Geometry check sheet. Reference: the model listing, model coordinates, mm. Round coordinates to 2 decimals unless told otherwise and drop trailing zeros. Order: outer loops, then holes, each group sorted by start corner. A loop starts at its lowest first (then second) coordinate and runs counter-clockwise, first axis right, second up.
```python
from build123d import *

# Parameters (mm, degrees)
F1_DEPTH = 3.81
F2_R     = 5.9944
F3_DEPTH = 25.4
F4_R     = 25.4


with BuildPart() as f1:
    # F0 (on Front) → F1 (new body)
    with BuildSketch(Plane.XZ):
        with BuildLine():
            ThreePointArc((-77.47, 0), (-76.2, 1.27), (-74.93, 0))
            Line((-74.93, 0), (-1.27, 0))
            ThreePointArc((-1.27, 0), (0, 1.27), (1.27, 0))
            Line((1.27, 0), (12.7, 0))
            Line((12.7, 0), (12.7, 12.7))
            Line((12.7, 12.7), (-88.9, 12.7))
            Line((-88.9, 12.7), (-88.9, 0))
            Line((-88.9, 0), (-77.47, 0))
        make_face()
        with BuildLine():
            ThreePointArc((-76.2, -1.27), (-77.0980256121, -0.8980256121), (-77.47, 0))
            Line((-77.47, 0), (-88.9, 0))
            Line((-88.9, 0), (-88.9, -76.2))
            Line((-88.9, -76.2), (-76.2, -76.2))
            Line((-76.2, -76.2), (-76.2, -1.27))
        make_face()
        with BuildLine():
            Line((-1.27, 0), (-74.93, 0))
            ThreePointArc((-74.93, 0), (-75.3019743879, -0.8980256121), (-76.2, -1.27))
            Line((-76.2, -1.27), (-76.2, -76.2))
            Line((-76.2, -76.2), (-69.85, -76.2))
            Line((-69.85, -76.2), (-6.35, -76.2))
            Line((-6.35, -76.2), (-6.35, -71.12))
            ThreePointArc((-6.35, -71.12), (-7.2480256121, -68.9519743879), (-5.08, -69.85))
            Line((-5.08, -69.85), (0, -69.85))
            Line((0, -69.85), (0, -1.27))
            ThreePointArc((0, -1.27), (-0.8980256121, -0.8980256121), (-1.27, 0))
        make_face()
        with BuildLine():
            ThreePointArc((-68.58, -69.85), (-68.9519743879, -70.7480256121), (-69.85, -71.12))
            ThreePointArc((-69.85, -71.12), (-70.7480256121, -68.9519743879), (-68.58, -69.85))
        make_face(mode=Mode.SUBTRACT)
        with BuildLine():
            Line((0, -76.2), (0, -69.85))
            Line((0, -69.85), (-5.08, -69.85))
            ThreePointArc((-5.08, -69.85), (-5.4519743879, -70.7480256121), (-6.35, -71.12))
            Line((-6.35, -71.12), (-6.35, -76.2))
            Line((-6.35, -76.2), (0, -76.2))
        make_face()
        with BuildLine():
            Line((12.7, 0), (1.27, 0))
            ThreePointArc((1.27, 0), (0.8980256121, -0.8980256121), (0, -1.27))
            Line((0, -1.27), (0, -69.85))
            Line((0, -69.85), (0, -76.2))
            Line((0, -76.2), (12.7, -76.2))
            Line((12.7, -76.2), (12.7, 0))
        make_face()
    extrude(amount=F1_DEPTH)

    # F2 (on face) → F3 (cut)
    with BuildSketch(Plane.XZ.offset(3.81)):
        with Locations((-70.104, -31.75)):
            Circle(F2_R)
        with BuildLine():
            Line((-38.1, -31.75), (-38.1, -25.7556))
            ThreePointArc((-38.1, -25.7556), (-42.3386808891, -27.5113191109), (-44.0944, -31.75))
            Line((-44.0944, -31.75), (-38.1, -31.75))
        make_face()
        with BuildLine():
            ThreePointArc((-32.1056, -31.75), (-33.8613191109, -27.5113191109), (-38.1, -25.7556))
            Line((-38.1, -25.7556), (-38.1, -31.75))
            Line((-38.1, -31.75), (-32.1056, -31.75))
        make_face()
        with BuildLine():
            Line((-32.1056, -31.75), (-38.1, -31.75))
            Line((-38.1, -31.75), (-44.0944, -31.75))
            ThreePointArc((-44.0944, -31.75), (-38.1, -37.7444), (-32.1056, -31.75))
        make_face()
        with BuildLine():
            ThreePointArc((-0.1016, -31.75), (-6.096, -25.7556), (-12.0904, -31.75))
            ThreePointArc((-12.0904, -31.75), (-6.096, -37.7444), (-0.1016, -31.75))
        make_face()
    extrude(amount=-F3_DEPTH, mode=Mode.SUBTRACT)

    # F4
    f4_edges = [f1.edges().sort_by_distance(p)[0] for p in [
        (12.7, -1.905, 12.7),
        (-88.9, -1.905, 12.7),
        (12.7, -1.905, -76.2),
        (-88.9, -1.905, -76.2),
    ]]
    fillet(f4_edges, radius=F4_R)


solid = f1.part
```
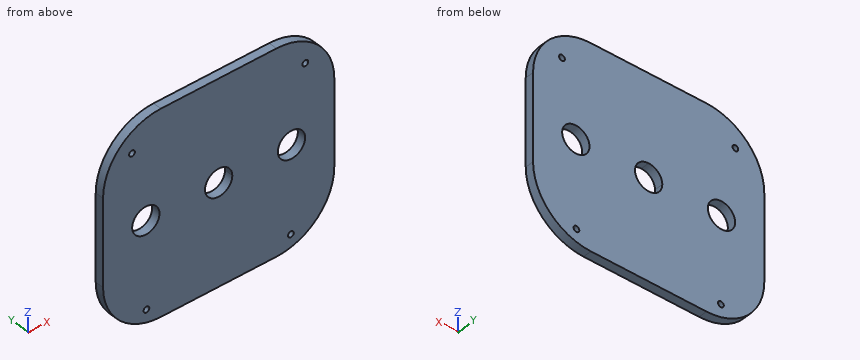
(1) Sectioned sample at A-A, the plane x = -43. Record the cut outline in (y, z), and give its area (3 significant figures).
Returned:
outline: (-3.81, -76.2) - (0, -76.2) - (0, -35.2) - (-3.81, -35.2) - close; (-3.81, -28.3) - (0, -28.3) - (0, 12.7) - (-3.81, 12.7) - close
area: 312 mm2
(2) Material ranges on line 1 (Z direction, x = -69.85, y = -2.4); line 2 (X direction, y = -2.2, z = -35.5); line 3 (X direction, y = -2.15, z = -69.85), recorded low to high.
Returned:
line 1: z = -75.39 to -71.12, -68.58 to -37.74, -25.76 to 11.89
line 2: x = -88.9 to -74.78, -65.43 to -42.78, -33.42 to -10.77, -1.42 to 12.7
line 3: x = -80.3 to -71.12, -68.58 to -7.62, -5.08 to 4.1
(3) Depth check by flat-ended pin: P1, Ø7, axis at x = -70.104, z = -31.75, coming from the +Y side; P2, Ø5, axis at x = -62.5, z = -55, coming from the +Y side. Enter the tip coordinate at first touch or a pass-through.
Returned:
P1: passes through
P2: stops at y = 0
(4) Sectioned sample at D-D, the plane z = 3.5. Record the cut outline in (x, y), and give its area (3 significant figures).
Returned:
outline: (-83.06, -3.81) - (6.86, -3.81) - (6.86, 0) - (-83.06, 0) - close
area: 343 mm2
(5) Sectioned sample at B-B, the plane y = -2.5. Record the cut outline in (x, z), and give its area (3 significant figures).
Returned:
outline: (-88.9, -50.8) arc R25.4 ccw to (-63.5, -76.2) - (-12.7, -76.2) arc R25.4 ccw to (12.7, -50.8) - (12.7, -12.7) arc R25.4 ccw to (-12.7, 12.7) - (-63.5, 12.7) arc R25.4 ccw to (-88.9, -12.7) - close; hole circle Ø2.54 at (-76.2, 0); hole circle Ø11.99 at (-70.1, -31.75); hole circle Ø2.54 at (-69.85, -69.85); hole circle Ø11.99 at (-38.1, -31.75); hole circle Ø11.99 at (-6.1, -31.75); hole circle Ø2.54 at (-6.35, -69.85); hole circle Ø2.54 at (0, 0)
area: 8,120 mm2
(6) Sectioned sample at C-C, the plane z = -29. Record the cut outline in (x, y).
Returned:
outline: (-88.9, -3.81) - (-75.43, -3.81) - (-75.43, 0) - (-88.9, 0) - close; (-64.78, -3.81) - (-43.43, -3.81) - (-43.43, 0) - (-64.78, 0) - close; (-32.77, -3.81) - (-11.42, -3.81) - (-11.42, 0) - (-32.77, 0) - close; (-0.77, -3.81) - (12.7, -3.81) - (12.7, 0) - (-0.77, 0) - close
